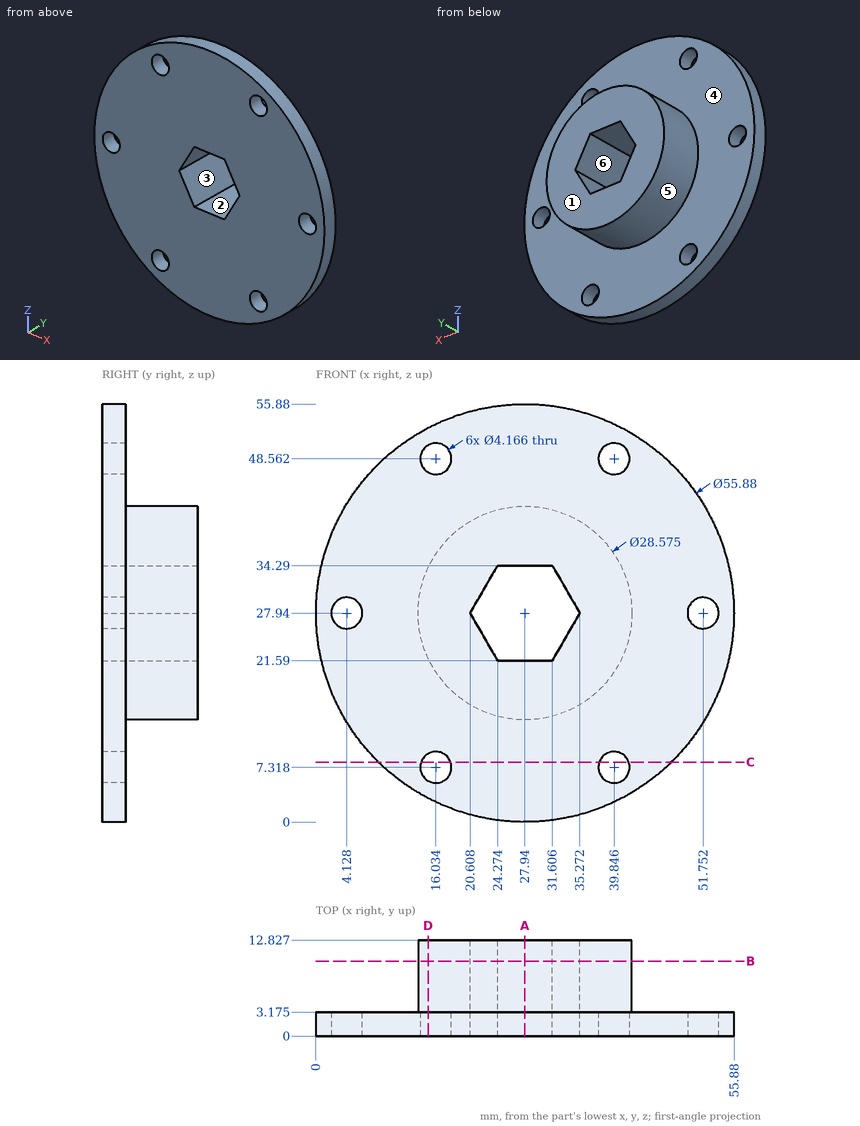
Design review of the part shown in the three views and the two pictorial views. Dimensions are in mm from the part's minimum x, y and z. A direction names the side the tool comes from. Round coordinates to 2 decimals unless told otherwise and drop trailing zeros. Order: outer loops, then holes, each group sorted by start corner. A loop starts at its lowest first (then second) coordinate and runs counter-clockwise, first axis right, second up. Notation, with made-up numbers: (-39.5, -40) - (19.5, -40) arc R15 ccw to (19.5, -34) - close; hole circle Ø2 at (50.25, 14.5). An arc over 180 degrees is marked (long way). One line per question, with ' | ' between items.
Item 1: Take a section at B-B, the plane y = 10. Write out the cut boundary in (x, z) (1 decimal).
Checks:
outline: circle Ø28.6 at (27.9, 27.9); hole (20.6, 27.9) - (24.3, 21.6) - (31.6, 21.6) - (35.3, 27.9) - (31.6, 34.3) - (24.3, 34.3) - close
Item 2: Machinability: for the marked faces 1 and 2, which of the approach directions +Z, -Z, +X, -X, +Y, -Y give a long, thin tool a straight path to every point of the face, cutting with its end or side? Answer none if there is none.
Checks:
face 1: +Z, -Z, +X, -X, +Y | face 2: +Y, -Y
Item 3: For P1, Ø5.5, axis at x = 16.03, z = 48.56, coming from the +Y side (1 decimal); P2, Ø6, axis at x = 26.5, y = 5.5, coming from the +Z side; P3, Ø2, axis at x = 14.5, y = 8, coming from the +Z side (1 decimal); P4, Ø6.5, axis at x = 51.75, z = 27.94, coming from the -Y side, all flat-tipped, find the tip position at first contact; note any pin that passes through.
Checks:
P1: y = 3.2 | P2: z = 55.88 | P3: z = 35 | P4: y = 0
Item 4: Draft analysis for pull direction X (two halves, no side actions). For the marked faces 3, 4, 5 and 6, state which applies: +X half, -X half, draft (parallel to the pull), parting line (faces both ways), or undercut.
Checks:
face 3: undercut | face 4: draft | face 5: parting line | face 6: undercut
Item 5: Take a section at A-A, the plane x = 27.94. Write out the cut boundary in (y, z) (1 decimal).
Checks:
outline: (0, 0) - (3.2, 0) - (3.2, 13.7) - (12.8, 13.7) - (12.8, 21.6) - (0, 21.6) - close; (0, 34.3) - (12.8, 34.3) - (12.8, 42.2) - (3.2, 42.2) - (3.2, 55.9) - (0, 55.9) - close
Item 6: Take a section at C-C, the plane z = 8. Write out the cut boundary in (x, y) (1 decimal).
Checks:
outline: (8.4, 0) - (14.1, 0) - (14.1, 3.2) - (8.4, 3.2) - close; (18, 0) - (37.9, 0) - (37.9, 3.2) - (18, 3.2) - close; (41.8, 0) - (47.5, 0) - (47.5, 3.2) - (41.8, 3.2) - close
Item 7: Take a section at D-D, the plane x = 15. Write out the cut boundary in (y, z) (1 decimal), then the cut area to 3 significant figures.
Checks:
outline: (0, 3.2) - (3.2, 3.2) - (3.2, 5.5) - (0, 5.5) - close; (0, 9.1) - (3.2, 9.1) - (3.2, 21.9) - (12.8, 21.9) - (12.8, 34) - (3.2, 34) - (3.2, 46.8) - (0, 46.8) - close; (0, 50.4) - (3.2, 50.4) - (3.2, 52.7) - (0, 52.7) - close | area: 251 mm²
Item 8: Wall thickness on line 1 (X direction, y = 1.25, z = 49.5) (1 decimal); line 2 (Y direction, x = 23, z = 45) (1 decimal); line 3 (X direction, y = 4.5, z = 22) (1 decimal): over which ranges is each line inside the solid? List them lowest first. Write a range as [from, to].
Checks:
line 1: [10.2, 14.2], [17.9, 38], [41.7, 45.7] | line 2: [0, 3.2] | line 3: [14.9, 24], [31.8, 40.9]
